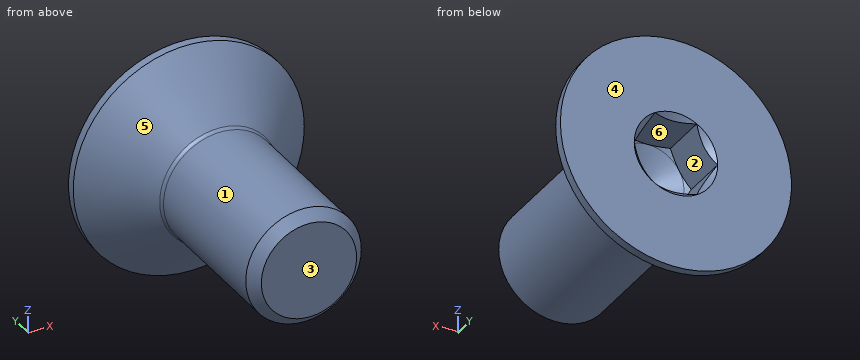
from build123d import *

# Parameters (mm, degrees)
CORTE_EXTRUS_O1_REACH = 11.798


with BuildPart() as part:
    # Esboço1 → Revolução1 (revolve)
    with BuildSketch(Plane.XY):
        with BuildLine():
            Line((0, -2.551075774), (1.25, -1.8))
            Line((1.25, -1.8), (1.25, 0))
            Line((1.25, 0), (4, 0))
            Line((4, 0), (4, -0.3))
            Line((4, -0.3), (2.058578644, -2.241421356))
            ThreePointArc((2.058578644, -2.241421356), (2.015224094, -2.306306026), (2, -2.382842712))
            Line((2, -2.382842712), (2, -7.65))
            Line((2, -7.65), (1.65, -8))
            Line((1.65, -8), (0, -8))
            Line((0, -8), (0, -2.551075774))
        make_face()
    revolve(axis=Axis((0, -1000, 0), (0, 1, 0)))

    # Corte-extrusão1: up to this cone (the profile starts inside it)
    corte_extrus_o1_end = Plane(origin=(0, 0, 0), z_dir=(0, 1, 0)).offset(-2.551074774) * Cone(1.664e-06, 31.779048647, 19.094777842, align=(Align.CENTER, Align.CENTER, Align.MIN), mode=Mode.PRIVATE)
    # Esboço2 → Corte-extrusão1 (cut, up to the surface)
    with BuildSketch(Plane(origin=(0, 0, 0), x_dir=(1, 0, 0), z_dir=(0, 1, 0)), mode=Mode.PRIVATE) as corte_extrus_o1_sk1:
        Polygon((-1.443375673, 0), (-0.721687836, -1.25), (0.721687836, -1.25), (1.443375673, 0), (0.721687836, 1.25), (-0.721687836, 1.25), align=None)
    corte_extrus_o1_tool1 = extrude(corte_extrus_o1_sk1.sketch, amount=-CORTE_EXTRUS_O1_REACH, mode=Mode.PRIVATE) & corte_extrus_o1_end
    add(corte_extrus_o1_tool1.solids().sort_by_distance((0, 0, 0))[0], mode=Mode.SUBTRACT)

    # Esboço3 → Corte-Revolução1 (revolve, cut)
    with BuildSketch(Plane.XY, mode=Mode.PRIVATE) as corte_revolu_o1_sk:
        Polygon((1.443375673, 0), (0, -1.443375673), (0, 0), align=None)
    revolve(corte_revolu_o1_sk.sketch.rotate(Axis((0, -1000, 0), (0, 1, 0)), 180), axis=Axis((0, -1000, 0), (0, 1, 0)), mode=Mode.SUBTRACT)


solid = part.part
Source: CAD feature listing. Evaluate the final solid. Frame: model axes, mm. Face numbers are marked on the shaded views. A direction names the side the tool comes from. Round coordinates to 2 decimals unless told otherwise and drop trailing zeros. Loops run counter-clockwise (first coordinate to the right, second up) from the corner with the lowest first, then second, coordinate; pieces in that order, holes last. Notation, with made-up numbers: (-21.5, -1) -> (-14.5, -1) arc R21 ccw to (-14.5, 14) -> close; hole circle Ø5 at (87.25, 30.25). An arc over 180 degrees is marked (long way). Answer as a JSON object with one key per item and string values. Group by question number.
Q1. Access query for the marked faces 1, 2 and 3. Directions: +Z, -Z, +X, -X, +Y, -Y. A direction counts if a zero-diameter tool reaches every point of the face in a straight line with its end or side. Return the directions, or none.
Q2. Contact query for flat-ended pins moving along their axis: P1, Ø4, axis at x = 0, z = -2, coming from the -Y side; P2, Ø1.5, axis at y = -5.5, z = 3, coming from the +X side; P3, Ø2, axis at x = 1, y = -1.5, coming from the +Z side; P4, Ø1.5, axis at x = 2, y = -1, coming from the -Z side. Output: stop coordinate, or through.
Q3. Section query A-A (y = -1.5). Output: boundary loops of the cut face in (x, z), plus the area to 3 significant figures.
Q4. Mould query, pull axis Z, two halves, no side actions, for the marked faces 4, 5 and 6. Classes: pulls with the +Z half, pulls with the -Z half, needs draft (parallel to the pull), parting line crosses it, or undercut.
Q5. Section query B-B (y = -6.5). Output: boundary loops of the cut face in (x, z).
Q6. Ray query, line 1 (Y direction, x = -2, z = 1.5); line 2 (Y direction, x = 0.75, z = 3.5); line 3 (X direction, y = -3, z = 0). Return the intervals inside material, ascending. Write a range as from..to.
Completed:
{
 "1": {"face 1": "-Y", "face 2": "+Y", "face 3": "+Z, -Z, +X, -X, -Y"},
 "2": {"P1": "y = -8", "P2": "through", "P3": "z = 3.69", "P4": "z = -3.61"},
 "3": {"outline": "circle Ø5.6 at (0, 0); hole (-1.44, 0) -> (-0.72, -1.25) -> (0.72, -1.25) -> (1.44, 0) -> (0.72, 1.25) -> (-0.72, 1.25) -> close", "area": "19.2 mm²"},
 "4": {"face 4": "needs draft", "face 5": "parting line crosses it", "face 6": "undercut"},
 "5": {"outline": "circle Ø4 at (0, 0)"},
 "6": {"line 1": "-1.8..0", "line 2": "-0.72..0", "line 3": "-2..2"}
}
